Input: part model. Units: mm. Frame: model coordinates. Face numbers are marked on the shaded views. A direction names the side the tool comes from. Give positions to 0.01 mm unless a question says otherwise; leave off trailing zeros. Write each loop counter-clockwise with the first axis right and the second up, starting at its lowest first coordinate (ties: lowest second). Pieces come first, ordered by that corner, then holes. Notation, with made-up numbers: (68.25, 27) -> (85.25, 27) arc R28 ccw to (85.25, 49) -> close; hole circle Ø10 at (11, 85.5). An arc over 180 degrees is marked (long way). Return JSON: item names as keys, results as strings. Group by question number.
Item 1: Section A-A, the plane z = -13. Return loops of the section in (x, y), then the cut area to 3 significant figures.
Item 2: Mould query, pull axis X, two halves, no side actions, for the marked faces 1 and 2. Classes: released by +X, released by -X, zero draft, split by the parting line, or undercut.
Item 3: Line query: line 1 (Y direction, x = -11.5, z = 16); line 2 (Z direction, x = -1.5, y = 35). Output: solid intervals per line, ascending. Write a range as [from, to].
Item 4: Set-up query: the marked faces 3, 4, 5 and 6. Return all of +Z, -Z, +X, -X, +Y, -Y with unobstructed straight access to the full face (end or side cutting, diameter ignored); none if empty.
Item 5: Pin query (flat end, axial travel): P1, Ø8, axis at x = -13.5, y = 1, coming from the +Z side (3 decimals); P2, Ø5.5, axis at x = 30.5, z = 19, coming from the +Y side; P3, Ø12, axis at y = 8.5, z = 4, coming from the +X side. Return the tip coordinate at first contact, or that it passes through.
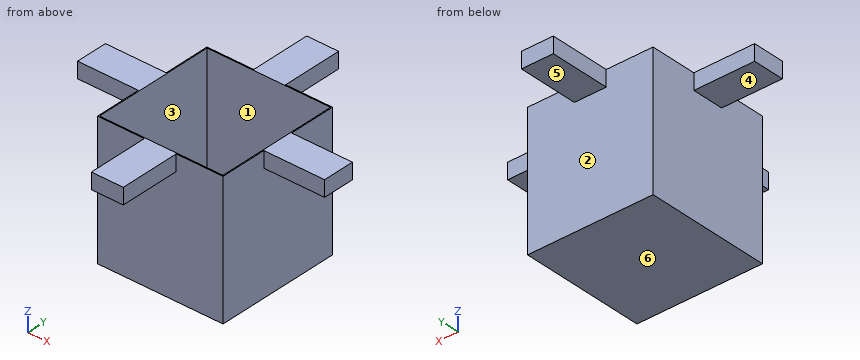
from build123d import *

# Parameters (mm, degrees)
F0_W      = 40
F0_H      = 42.5
F1_DEPTH  = 20
F2_W      = 39.365
F2_H      = 39.365
F3_DEPTH  = 41.865
F4_W      = 10.16
F4_H      = 5.08
F8_DEPTH  = 19.365
F5_W      = 10.16
F5_H      = 5.08
F9_DEPTH  = 19.365
F6_W      = 10.16
F6_H      = 5.08
F10_DEPTH = 19.365
F7_W      = 10.16
F7_H      = 5.08
F11_DEPTH = 19.365


with BuildPart() as f1:
    # F0 (on Front) → F1 (new body, symmetric)
    with BuildSketch(Plane.XZ):
        Rectangle(F0_W, F0_H)
    extrude(amount=F1_DEPTH, both=True)

    # F2 (on face) → F3 (cut)
    with BuildSketch(Plane.XY.offset(21.25)):
        Rectangle(F2_W, F2_H)
    extrude(amount=-F3_DEPTH, mode=Mode.SUBTRACT)

    # F4 (on face) → F8 (join)
    with BuildSketch(Plane.XZ.offset(20)):
        with Locations((0, 18.71)):
            Rectangle(F4_W, F4_H)
    extrude(amount=F8_DEPTH)

    # F5 (on face) → F9 (join)
    with BuildSketch(Plane(origin=(-20, 0, 0), x_dir=(0, -1, 0), z_dir=(-1, 0, 0))):
        with Locations((0, 18.71)):
            Rectangle(F5_W, F5_H)
    extrude(amount=F9_DEPTH)

    # F6 (on face) → F10 (join)
    with BuildSketch(Plane(origin=(0, 20, 0), x_dir=(-1, 0, 0), z_dir=(0, 1, 0))):
        with Locations((0, 18.71)):
            Rectangle(F6_W, F6_H)
    extrude(amount=F10_DEPTH)

    # F7 (on face) → F11 (join)
    with BuildSketch(Plane.YZ.offset(20)):
        with Locations((0, 18.71)):
            Rectangle(F7_W, F7_H)
    extrude(amount=F11_DEPTH)


solid = f1.part
Answer below:
{
 "1": {"outline": "(-20, -20) -> (20, -20) -> (20, 20) -> (-20, 20) -> close; hole (-19.68, -19.68) -> (19.68, -19.68) -> (19.68, 19.68) -> (-19.68, 19.68) -> close", "area": "50.4 mm2"},
 "2": {"face 1": "undercut", "face 2": "zero draft"},
 "3": {"line 1": "y = [-20, -19.68], [19.68, 20]", "line 2": "z = [16.17, 21.25]"},
 "4": {"face 3": "+Z", "face 4": "-Z, -X, +Y, -Y", "face 5": "-Z, +X, -X, +Y", "face 6": "-Z, +X, -X, +Y, -Y"},
 "5": {"P1": "stops at z = -20.615", "P2": "stops at y = 5.08", "P3": "stops at x = 20"}
}
